Autodesk Fusion 360 part; units mm, degrees
sketch "Sketch1" plane through (0, 0, 0) normal (0, 0, 1) x (1, 0, 0) in component "Holder"
  line L0 (0, 0) -> (30, 0)
  line L1 (30, 0) -> (30, 30)
  line L2 (30, 30) -> (0, 30)
  line L3 (0, 30) -> (0, 0)
  circle A0 centre (5, 25) radius 2
  circle A1 centre (5, 5) radius 2
  circle A2 centre (25, 25) radius 2
  circle A3 centre (25, 5) radius 2
  dimension "d1" = 30
  dimension "d2" = 30
  dimension "d4" = 4
  dimension "d5" = 4
  dimension "d6" = 20
  dimension "d7" = 5
  dimension "d8" = 5
  dimension "d9" = 4
  dimension "d10" = 20
  dimension "d11" = 5
  dimension "d12" = 4
  dimension "d13" = 20
  dimension "d14" = 20
extrude "Extrude1" add sketch "Sketch1" along normal blind 5 in component "Holder"
sketch "Sketch2" plane through (0, 0, 5) normal (0, 0, 1) x (-1, 0, 0) in component "Holder"
  circle A0 centre (-5, -5) radius 2
  circle A1 centre (-25, -5) radius 2
  circle A2 centre (-5, -25) radius 2
  circle A3 centre (-25, -25) radius 2
  line L0 (0, -30) -> (0, 0)
  line L1 (0, 0) -> (-30, 0)
  line L2 (-30, 0) -> (-30, -30)
  line L3 (-30, -30) -> (0, -30)
  line L4 (-7.5, -22.5) -> (-22.5, -22.5)
  line L5 (-22.5, -22.5) -> (-22.5, -7.5)
  line L6 (-22.5, -7.5) -> (-7.5, -7.5)
  line L7 (-7.5, -7.5) -> (-7.5, -22.5)
  circle A4 centre (-15, -15) radius 5.9
  dimension "d17" = 15
  dimension "d18" = 15
  dimension "d19" = 7.5
  dimension "d20" = 7.5
  dimension "d21" = 11.8
  dimension "d22" = 15
extrude "Extrude2" add sketch "Sketch2" along normal blind 30 contours L4 L5 L6 L7 in component "Holder"
extrude "Extrude3" add 1 faces at (15.147, 8.0388, 35) along direction (0, 0, 1) blind 2 in component "Holder"
extrude "Extrude4" add 1 faces at (15.147, 8.0388, 37) along direction (0, 0, 1) blind 18 in component "Holder"
extrude "Extrude5" add 1 faces at (15.147, 8.0388, 55) along direction (0, 0, 1) blind 180 in component "Holder"
component "Holder" placed x (1, 0, 0) y (0, 1, 0) z (0, 0, 1) at (0, 0, 0)
Geometry check sheet. Reference: the model listing, model coordinates, mm. A direction names the side the tool comes from. Round coordinates to 2 decimals unless told otherwise and drop trailing zeros. Order: outer loops, then holes, each group sorted by start corner. A loop starts at its lowest first (then second) coordinate and runs counter-clockwise, first axis right, second up. Notation, with made-up numbers: M -9.75,14.5 L 31.25,14.5 A20 ccw 31.25,18.5 Z; hole C -22,32 d9. An arc over 180 degrees is marked long. Answer in a Markdown table with one row per item. Add a question column.
Item 1: Set-up check for faces 4 (the face through (15, 22.5, 118)), 5 (the face through (15, 15, 5)), 6 (the face through (15, 30, 2)), 7 (the face through (22.5, 15, 118)), 8 (the face through (30, 15, 2)): record each of +Z, -Z, +X, -X, +Y, -Y from which the full face is reachable in a straight line by a thin tool's end or side.
Item 2: Depth check by flat-ended pin: pin 1 Ø16.5 at (x, z) = (12.5, 156) entering from +Y; pin 2 Ø12 at (y, z) = (15, 135) entering from +X; pin 3 Ø3 at (x, y) = (5, 5) entering from -Z; pin 4 Ø1.5 at (x, z) = (20.5, 84) entering from -Y. Enter the tip coordinate at first touch or a pass-through.
Item 3: Sectioned sample at D-D, the plane x = 15. Enter the section's corners in (y, z).
Item 4: Draft check along Y on faces 1 (the face through (3.4, 6.2, 2.5)), 2 (the face through (7.5, 15, 118)), 3 (the face through (15, 7.5, 118)). Enter one of: released by +Y, released by -Y, zero draft, split by the parting line, or undercut.
Item 5: Sectioned sample at A-A, the plane x = 5. Enter the section's corners in (y, z).
Item 6: Sectioned sample at B-B, the plane z = 51. Enter the section's corners in (x, y).
Item 7: Material ranges on L1, parallel to Y at x = 25, z = 1.65; L2, parallel to Y at x = 15, z = 133, recorded low to high. Write a range as [from, to].
Filled in:
| question | item | result |
|---|---|---|
| 1 | face 4 | +Z, +X, -X, +Y |
| 1 | face 5 | +Z |
| 1 | face 6 | +Z, -Z, +X, -X, +Y |
| 1 | face 7 | +Z, +X, +Y, -Y |
| 1 | face 8 | +Z, -Z, +X, +Y, -Y |
| 2 | pin 1 | stops at y = 22.5 |
| 2 | pin 2 | stops at x = 22.5 |
| 2 | pin 3 | passes through |
| 2 | pin 4 | stops at y = 7.5 |
| 3 | outline | M 0,0 L 30,0 L 30,5 L 22.5,5 L 22.5,235 L 20.9,235 L 20.9,5 L 9.1,5 L 9.1,235 L 7.5,235 L 7.5,5 L 0,5 Z |
| 4 | face 1 | undercut |
| 4 | face 2 | zero draft |
| 4 | face 3 | released by -Y |
| 5 | outline | M 0,0 L 3,0 L 3,5 L 0,5 Z; M 7,0 L 23,0 L 23,5 L 7,5 Z; M 27,0 L 30,0 L 30,5 L 27,5 Z |
| 6 | outline | M 7.5,7.5 L 22.5,7.5 L 22.5,22.5 L 7.5,22.5 Z; hole C 15,15 d11.8 |
| 7 | L1 | y = [0, 3], [7, 23], [27, 30] |
| 7 | L2 | y = [7.5, 9.1], [20.9, 22.5] |
